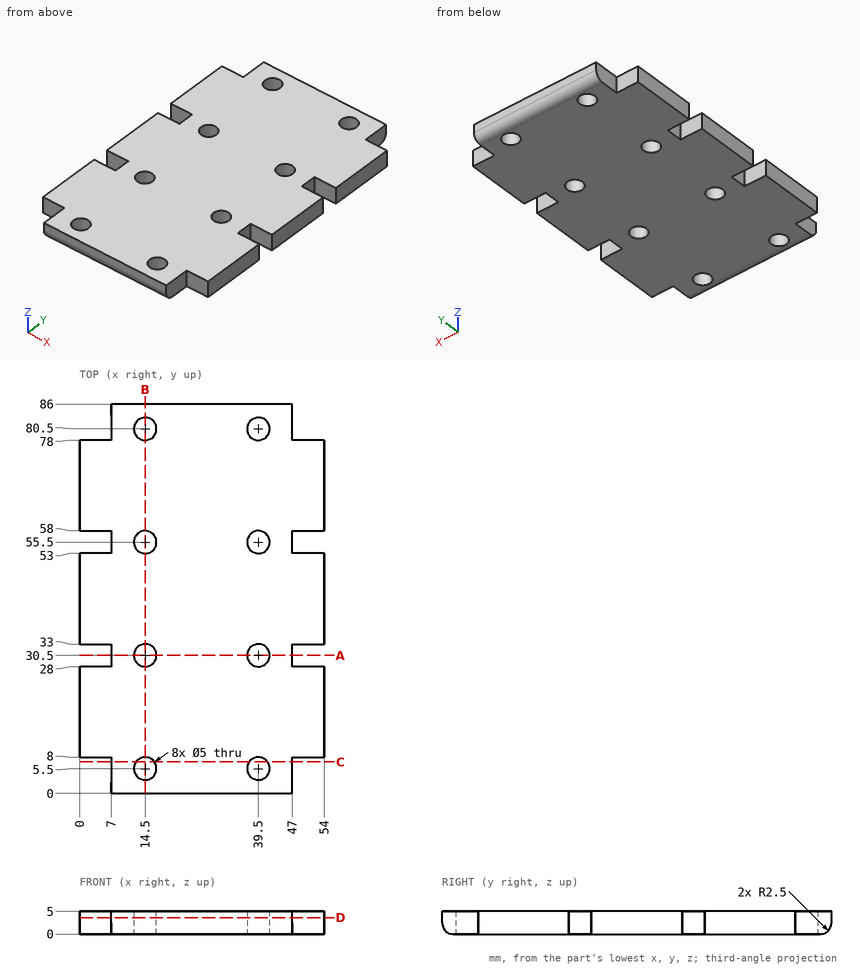
The figure shows three views and two pictorial views of one solid part (mm, origin at its lowest corner). Answer the questions. Coordinates: 2 decimals unless noted, no trailing zeros. Loops run counter-clockwise (first coordinate to the right, second up) from the corner with the lowest first, then second, coordinate; pieces in that order, holes last.
1) Find section D-D on z = 3.65. Give the number of separate pieces and of enclosed holes in the cut face, then the cut area to 3 significant figures.
2) Find section B-B on x = 14.5. Write down the section's boundary in (y, z), then the cut area to 3 significant figures.
3) Find section A-A on y = 30.5. Write down the section's boundary in (x, z).
4) Find section C-C on y = 7. Write down the section's boundary in (x, z), then the cut area to 3 significant figures.
5) Flat-ended cylindrical pins translate along their axes: pin 1 Ø1.5 at (x, z) = (50, 1.5) entering from +Y; pin 2 Ø3 at (x, z) = (15.5, 4.5) entering from -Y; pin 3 Ø1.5 at (y, z) = (83.5, 1.5) entering from -X; pin 4 Ø3 at (x, y) = (14.5, 80.5) entering from -Z. Find the tip coordinate at first contact, or state that the pin passes through.
6) Find the intervals of material crossed by L1, parallel to Y at x = 14.5, z = 1.2; L2, parallel to Y at x = 14.5, z = 1.7; L3, parallel to X at y = 29, z = 2.2, in increasing order.
Values:
1. separate pieces: 1
1. enclosed holes: 8
1. area: 4,120 mm2
2. outline: (0, 2.5) arc R2.5 ccw to (2.5, 0) - (3, 0) - (3, 5) - (0, 5) - close; (8, 0) - (28, 0) - (28, 5) - (8, 5) - close; (33, 0) - (53, 0) - (53, 5) - (33, 5) - close; (58, 0) - (78, 0) - (78, 5) - (58, 5) - close; (83, 0) - (83.5, 0) arc R2.5 ccw to (86, 2.5) - (86, 5) - (83, 5) - close
2. area: 327 mm2
3. outline: (7, 0) - (12, 0) - (12, 5) - (7, 5) - close; (17, 0) - (37, 0) - (37, 5) - (17, 5) - close; (42, 0) - (47, 0) - (47, 5) - (42, 5) - close
4. outline: (7, 0) - (12.5, 0) - (12.5, 5) - (7, 5) - close; (16.5, 0) - (37.5, 0) - (37.5, 5) - (16.5, 5) - close; (41.5, 0) - (47, 0) - (47, 5) - (41.5, 5) - close
4. area: 160 mm2
5. pin 1: stops at y = 78
5. pin 2: stops at y = 0
5. pin 3: stops at x = 7
5. pin 4: passes through
6. L1: y = 0.36 to 3, 8 to 28, 33 to 53, 58 to 78, 83 to 85.64
6. L2: y = 0.13 to 3, 8 to 28, 33 to 53, 58 to 78, 83 to 85.87
6. L3: x = 7 to 12.5, 16.5 to 37.5, 41.5 to 47
